Work out the finished part from the listing and answer in its coordinate system (mm). A direction names the side the tool comes from. Coordinates: 2 decimals unless noted, no trailing zeros. Order: outer loops, then holes, each group sorted by start corner. A loop starts at its lowest first (then second) coordinate and runs counter-clockwise, first axis right, second up. Notation, with made-up numbers: M -12.5,-38 L 41.5,-38 A24 ccw 41.5,-1 Z; hole C -37,19.25 d5. An arc over 180 degrees is marked long. Write item = value, one per line. Start each with the question number.
Q1. Straight lines are drawn through the part: line 1 along Y through (x, z) = (-2.75, 10); line 2 along Y through (x, z) = (-1.75, 10.75); line 3 along Y through (x, z) = (0, 2.5). For each, find the intervals that lie inside material, in ascending order.
Q2. Find section A-A on y = 0. Give the vertices of the cut face in (x, z), and give its area (3 significant figures).
Q3. Find section B-B on x = 0. Give the vertices of the cut face in (y, z).
Q4. Find section D-D on x = -5.75. Give the vertices of the cut face in (y, z).
Q5. Determine the mould class of faces 3 (the cylindrical face through (8.584, -2.703, 9.212)), 4 (the flat face through (2, -9, 6.5)), 5 (the cylindrical face through (-6.6, -2, 3.3)) for opening direction Y: released by +Y, released by -Y, zero draft, split by the parting line, or undercut.
Q6. Each of these flat-tipped pins is pushed along its axis until it touches: P1, Ø6, axis at x = -5.5, z = 8, coming from the -Y side; P2, Ø3, axis at x = -4, z = 7, coming from the -Y side; P3, Ø1.5, axis at x = 8.5, z = 4, coming from the -Y side; P4, Ø1.5, axis at x = 1, y = -0.5, coming from the +Z side. Where does it stop, or does it pass through?
Q7. A tool of negligible diameter and unlimited length cuts with its end or side. For faces 1 (the flat face through (2.3, -2.3, 0)), 2 (the cylindrical face through (-5.571, 0.923, 7.476)), from which of +Z, -Z, +X, -X, +Y, -Y can it reach the whole face along a straight path? Write none if from no direction.
Q8. Find section C-C on z = 10.25. Give the vertices of the cut face in (x, y).
Autodesk Inventor part; units mm, degrees
ref_plane "YZ Plane" through (0, 0, 0) normal (1, 0, 0) x (0, 1, 0)
ref_plane "XZ Plane" through (0, 0, 0) normal (0, 1, 0) x (-1, 0, 0)
ref_plane "XY Plane" through (0, 0, 0) normal (0, 0, 1) x (1, 0, 0)
sketch "Sketch3" plane through (0, 0, 0) normal (0, 0, 1) x (1, 0, 0)
  circle A0 centre (0, 0) radius 11
  circle A1 centre (0, 0) radius 3
  circle A2 centre (6.2, 0) radius 1.5
  circle A3 centre (3.1, 5.3694) radius 1.5
  circle A4 centre (-3.1, 5.3694) radius 1.5
  circle A5 centre (-6.2, 0) radius 1.5
  circle A6 centre (-3.1, -5.3694) radius 1.5
  circle A7 centre (3.1, -5.3694) radius 1.5
  dimension "d0" = 22
  dimension "d1" = 6
  dimension "d4" = 3
  dimension "d5" = 6.2
  dimension "d12" = 360
extrude "Extrusion1" add sketch "Sketch3" along normal blind 6.5 contours A0 | A3 | A5 | A7
sketch "Sketch6" plane through (0, 0, 6.5) normal (0, 0, 1) x (1, 0, 0)
  circle A0 centre (0, 0) radius 3
  circle A1 centre (-3.1, -5.3694) radius 1.5
  circle A2 centre (-3.1, 5.3694) radius 1.5
  circle A3 centre (6.2, 0) radius 1.5
  circle A4 centre (0, 0) radius 11
  circle A5 centre (0, 0) radius 9
  dimension "d27" = 18
extrude "Extrusion4" add sketch "Sketch6" along normal blind 5.5 contours A5
sketch "Sketch7" plane through (0, 0, 0) normal (1, 0, 0) x (0, 1, 0)
  circle A0 centre (0, 3.25) radius 2
  circle A1 centre (0, 9.25) radius 2
  line L0 (11, 0) -> (11, 6.5)
  line L1 (9, 6.5) -> (9, 12)
  point P0 (0, 0)
  point P1 (11, 3.25)
  point P2 (9, 9.25)
  dimension "d30" = 4
  dimension "d31" = 4
extrude "Extrusion5" cut sketch "Sketch7" against normal through all
thread "Thread5"
thread "Thread6"
thread "Thread7"
thread "Thread8"
thread "Thread9"
properties part number "6mm Mounting Hub, thin" material "ABS Plastic"
Findings below:
q1.line_1 = -8.57 to -6.83, -3.91 to -1.85, 1.85 to 3.91, 6.83 to 8.57
q1.line_2 = -8.83 to -6.02, -4.72 to -2.44, 2.44 to 4.72, 6.02 to 8.83
q1.line_3 = -11 to -3, 3 to 11
q2.outline = M -11,0 L -3,0 L -3,1.25 L -11,1.25 Z; M -11,5.25 L -3,5.25 L -3,7.25 L -9,7.25 L -9,6.5 L -11,6.5 Z; M -9,11.25 L -3,11.25 L -3,12 L -9,12 Z; M 3,0 L 4.7,0 L 4.7,12 L 3,12 Z; M 7.7,0 L 11,0 L 11,6.5 L 9,6.5 L 9,12 L 7.7,12 Z
q2.area = 78.0 mm^2
q3.outline = M -11,0 L -3,0 L -3,12 L -9,12 L -9,6.5 L -11,6.5 Z; M 3,0 L 11,0 L 11,6.5 L 9,6.5 L 9,12 L 3,12 Z
q4.outline = M -9.38,0 L 9.38,0 L 9.38,6.5 L 6.92,6.5 L 6.92,12 L -6.92,12 L -6.92,6.5 L -9.38,6.5 Z; hole C 0,3.25 d4; hole C 0,9.25 d4
q5.face_3 = split by the parting line
q5.face_4 = zero draft
q5.face_5 = undercut
q6.P1 = -10.61
q6.P2 = -10.69
q6.P3 = -7.81
q6.P4 = through
q7.face_1 = -Z, +X, -X, +Y, -Y
q7.face_2 = -X
q8.outline = M -8.83,-1.73 A9 ccw long -8.83,1.73 L -2.45,1.73 A3 cw long -2.45,-1.73 Z; hole C -3.1,-5.37 d3; hole C -3.1,5.37 d3; hole C 6.2,0 d3
